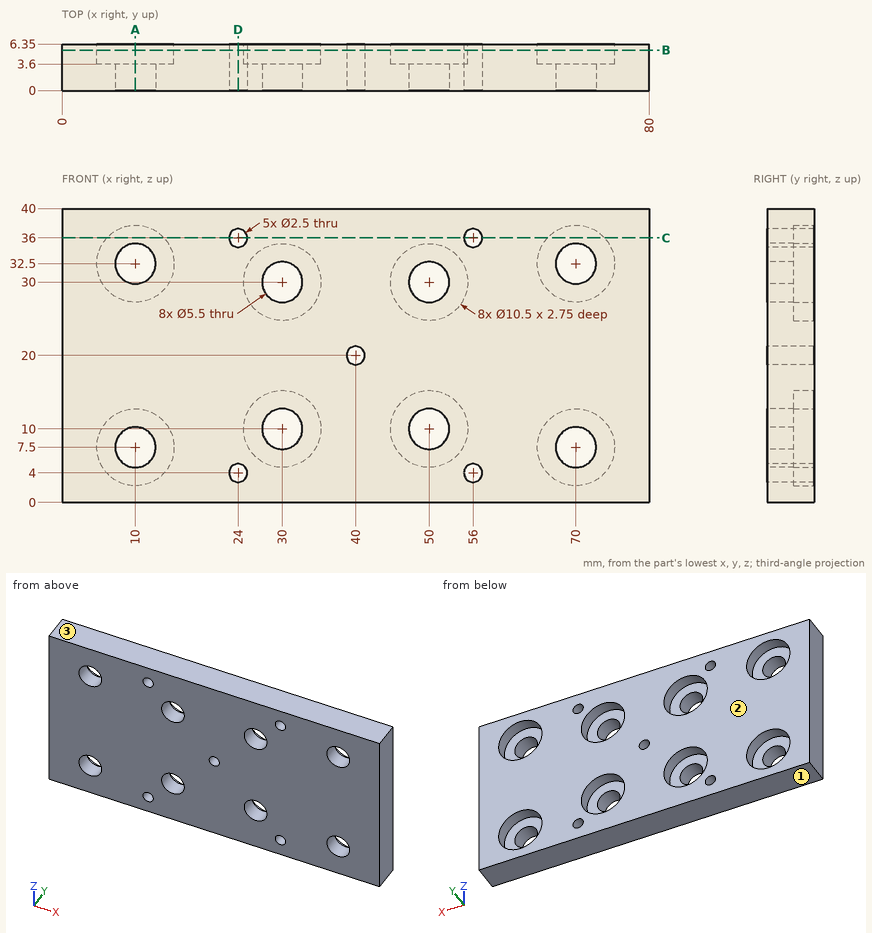
Geometry check sheet. Reference: drawing and pictorial views, mm from the part's lowest x, y, z. Coordinates: 2 decimals unless noted, no trailing zeros. Write each loop counter-clockwise with the first axis right and the second up, starting at its lowest first coordinate (ties: lowest second). Pieces come first, ordered by that corner, then holes. Notation, with made-up numbers: M 44.25,13 L 57.25,13 A22 ccw 57.25,50 Z; hole C 76.5,51.25 d8. An arc over 180 degrees is marked long. Write item = value, one per line. Start each with the question number.
1. Sectioned sample at D-D (x = 24). Record the cut outline in (y, z), then the cut area to 3 significant figures.
2. Go/stop test with flat-tipped pins: pin 1 (4.5 mm diameter, centred on x = 10, z = 7.5, fed in from +Y); pin 2 (5 mm diameter, centred on x = 48.5, z = 28.5, fed in from +Y). Record where each tip stops, or that it passes through.
3. Sectioned sample at C-C (z = 36). Record the cut outline in (x, y), then the cut area to 3 significant figures.
4. Sectioned sample at A-A (x = 10). Record the cut outline in (y, z), then the cut area to 3 significant figures.
5. Thickness scan on probe 1 along Z at (x, y) = (70, 2.6); probe 2 along X at (y, z) = (0.5, 11); probe 3 along Z at (x, y) = (40, 4.25). Record the ranges inside material, lowest first.
6. Mould release check, pull along Z, two halves, no side actions. Record for the marked faces 1, 2 and 3: pulls with the +Z half, pulls with the -Z half, needs draft (parallel to the pull), parting line crosses it, or undercut.
7. Sectioned sample at B-B (y = 5.5). State how many separate pieces and enclosed holes the cut face has, then the cut area to 3 significant figures.
The answers:
q1.outline = M 0,0 L 6.35,0 L 6.35,2.75 L 0,2.75 Z; M 0,5.25 L 6.35,5.25 L 6.35,34.75 L 0,34.75 Z; M 0,37.25 L 6.35,37.25 L 6.35,40 L 0,40 Z
q1.area = 222 mm²
q2.pin_1 = through
q2.pin_2 = 3.6
q3.outline = M 0,0 L 22.75,0 L 22.75,6.35 L 13.91,6.35 L 13.91,3.6 L 6.09,3.6 L 6.09,6.35 L 0,6.35 Z; M 25.25,0 L 54.75,0 L 54.75,6.35 L 25.25,6.35 Z; M 57.25,0 L 80,0 L 80,6.35 L 73.91,6.35 L 73.91,3.6 L 66.09,3.6 L 66.09,6.35 L 57.25,6.35 Z
q3.area = 433 mm²
q4.outline = M 0,0 L 6.35,0 L 6.35,2.25 L 3.6,2.25 L 3.6,4.75 L 0,4.75 Z; M 0,10.25 L 3.6,10.25 L 3.6,12.75 L 6.35,12.75 L 6.35,27.25 L 3.6,27.25 L 3.6,29.75 L 0,29.75 Z; M 0,35.25 L 3.6,35.25 L 3.6,37.75 L 6.35,37.75 L 6.35,40 L 0,40 Z
q4.area = 157 mm²
q5.probe_1 = 0 to 4.75, 10.25 to 29.75, 35.25 to 40
q5.probe_2 = 0 to 27.44, 32.56 to 47.44, 52.56 to 80
q5.probe_3 = 0 to 18.75, 21.25 to 40
q6.face_1 = pulls with the -Z half
q6.face_2 = needs draft
q6.face_3 = pulls with the +Z half
q7.separate_pieces = 1
q7.enclosed_holes = 13
q7.area = 2,480 mm²
